from build123d import *

# Parameters (mm, degrees)
SKETCH1_W           = 40
SKETCH1_H           = 40
BOSS_EXTRUDE1_DEPTH = 20
SKETCH2_R           = 3
BOSS_EXTRUDE2_DEPTH = 5
SKETCH3_W           = 20
SKETCH3_H           = 3
BOSS_EXTRUDE3_DEPTH = 7.5
SKETCH4_R           = 2.5
CUT_EXTRUDE1_DEPTH  = 7.5


with BuildPart() as part:
    # Sketch1 → Boss-Extrude1 (new body)
    with BuildSketch(Plane.XY):
        Rectangle(SKETCH1_W, SKETCH1_H)
    extrude(amount=BOSS_EXTRUDE1_DEPTH)

    # Sketch2 → Boss-Extrude2 (add)
    with BuildSketch(Plane(origin=(0, 20, 0), x_dir=(1, 0, 0), z_dir=(0, 1, 0))):
        with Locations(Location((9.5, -10, 0), (0, 0, 90))):
            Circle(SKETCH2_R)
    extrude(amount=BOSS_EXTRUDE2_DEPTH)

    # Sketch3 → Boss-Extrude3 (add)
    with BuildSketch(Plane.ZY.offset(20)):
        with Locations((10, 9.5)):
            Rectangle(SKETCH3_W, SKETCH3_H)
    boss_extrude3 = extrude(amount=BOSS_EXTRUDE3_DEPTH)

    # Sketch4 → Cut-Extrude1 (cut)
    with BuildSketch(Plane(origin=(0, 11, 0), x_dir=(1, 0, 0), z_dir=(0, 1, 0))):
        with Locations(Location((-23.75, -5, 0), (0, 0, 270))):
            Circle(SKETCH4_R)
        with Locations(Location((-23.75, -15, 0), (0, 0, 270))):
            Circle(SKETCH4_R)
    cut_extrude1 = extrude(amount=-CUT_EXTRUDE1_DEPTH, mode=Mode.SUBTRACT)

    # Mirror1: Boss-Extrude3, Cut-Extrude1 across plane
    add(boss_extrude3.mirror(Plane(origin=(0, 0, 0), x_dir=(0, 0, 1), z_dir=(1, 0, 0))))
    add(cut_extrude1.mirror(Plane(origin=(0, 0, 0), x_dir=(0, 0, 1), z_dir=(1, 0, 0))), mode=Mode.SUBTRACT)


solid = part.part
The listing builds one solid part. Answer for the finished solid, in the listing's coordinates (mm). A direction names the side the tool comes from. Coordinates: 2 decimals unless noted, no trailing zeros. Loops run counter-clockwise (first coordinate to the right, second up) from the corner with the lowest first, then second, coordinate; pieces in that order, holes last.
1) Find section B-B on x = -23.75. Write down the section's boundary in (y, z), then the cut area to 3 significant figures.
2) Find the intervals of material crossed by L1, parallel to Z at x = 23.75, y = 9.8; L2, parallel to X at y = 8.9, z = 5; L3, parallel to Z at x = 23, y = 9, in increasing order.
3) Flat-ended cylindrical pins translate along their axes: pin 1 Ø4 at (x, z) = (24.5, 6) entering from +Y; pin 2 Ø8 at (x, y) = (-8, 14) entering from -Z; pin 3 Ø4.5 at (y, z) = (15.5, 11.5) entering from +X; pin 4 Ø8 at (x, z) = (-12.5, 16) entering from +Y. Find the tip coordinate at first contact, or state that the pin passes through.
4) Find section C-C on x = 9.5. Write down the section's boundary in (y, z), then the cut area to 3 significant figures.
5) Find section D-D on z = 4.5. Write down the section's boundary in (x, y).
6) Find section A-A on z = 15. Write down the section's boundary in (x, y), then the cut area to 4 significant figures.
7) Determine the mould class of faces 6 (the face through (0, -20, 10)), 7 (the face through (-20, -6, 10)), 8 (the face through (27.5, 10, 10)), 9 (the face through (22.06, 9.52, 13.16)) for opening direction X: pulls with the +X half, pulls with the -X half, needs draft (parallel to the pull), parting line crosses it, or undercut.
8) A tool of negligible diameter and unlimited length cuts with its end or side. For faces 1 (the face through (7.47, 22.46, 12.21)), 2 (the face through (24, 8, 10)), 3 (the face through (-24, 8, 10)), 4 (the face through (20, 15, 10)), 5 (the face through (-24, 11, 10)), from which of +Z, -Z, +X, -X, +Y, -Y can it reach the whole face along a straight path? Write none if from no direction.
Values:
1. outline: (8, 0) - (11, 0) - (11, 2.5) - (8, 2.5) - close; (8, 7.5) - (11, 7.5) - (11, 12.5) - (8, 12.5) - close; (8, 17.5) - (11, 17.5) - (11, 20) - (8, 20) - close
1. area: 30.0 mm2
2. L1: z = 0 to 2.5, 7.5 to 12.5, 17.5 to 20
2. L2: x = -27.5 to -26.25, -21.25 to 21.25, 26.25 to 27.5
2. L3: z = 0 to 2.62, 7.38 to 12.62, 17.38 to 20
3. pin 1: stops at y = 11
3. pin 2: stops at z = 0
3. pin 3: stops at x = 20
3. pin 4: stops at y = 20
4. outline: (-20, 0) - (20, 0) - (20, 7) - (25, 7) - (25, 13) - (20, 13) - (20, 20) - (-20, 20) - close
4. area: 830 mm2
5. outline: (-27.5, 8) - (-26.2, 8) - (-26.2, 11) - (-27.5, 11) - close; (-21.3, 8) - (-20, 8) - (-20, -20) - (20, -20) - (20, 8) - (21.3, 8) - (21.3, 11) - (20, 11) - (20, 20) - (-20, 20) - (-20, 11) - (-21.3, 11) - close; (26.2, 8) - (27.5, 8) - (27.5, 11) - (26.2, 11) - close
6. outline: (-27.5, 8) - (-26.25, 8) - (-26.25, 11) - (-27.5, 11) - close; (-21.25, 8) - (-20, 8) - (-20, -20) - (20, -20) - (20, 8) - (21.25, 8) - (21.25, 11) - (20, 11) - (20, 20) - (-20, 20) - (-20, 11) - (-21.25, 11) - close; (26.25, 8) - (27.5, 8) - (27.5, 11) - (26.25, 11) - close
6. area: 1,615 mm2
7. face 6: needs draft
7. face 7: pulls with the -X half
7. face 8: pulls with the +X half
7. face 9: undercut
8. face 1: +Y
8. face 2: +Z, -Z, +X, -Y
8. face 3: +Z, -Z, -X, -Y
8. face 4: +Z, -Z, +X, +Y
8. face 5: +Z, -Z, -X, +Y
